from build123d import *

# Parameters (mm, degrees)
SKETCH064_R     = 1.9
POCKET002_DEPTH = 3
SKETCH065_R     = 2
POCKET003_DEPTH = 8


with BuildPart() as part:
    # Sketch063 → Revolution002 (revolve)
    with BuildSketch(Plane.XZ):
        Polygon((5, 13), (5, 0), (16, 0), (16, 3), (8, 3), (8, 13), align=None)
    revolve(axis=Axis((0, 0, 0), (0, 0, 1)))

    # Sketch064 → Pocket002 (cut)
    with BuildSketch(Plane.XY):
        with Locations((-8.485281, 8.485281)):
            Circle(SKETCH064_R)
        with Locations((8.485281, 8.485281)):
            Circle(SKETCH064_R)
        with Locations((8.485281, -8.485281)):
            Circle(SKETCH064_R)
        with Locations((-8.485281, -8.485281)):
            Circle(SKETCH064_R)
    extrude(amount=POCKET002_DEPTH, mode=Mode.SUBTRACT)

    # Sketch065 → Pocket003 (cut, symmetric)
    with BuildSketch(Plane.XZ):
        with Locations((0, 8)):
            Circle(SKETCH065_R)
    extrude(amount=POCKET003_DEPTH, both=True, mode=Mode.SUBTRACT)


with BuildPart() as part_1:
    # Body003 placement: moved
    add(part.part.moved(Location((0, 0, -54.75))))


solid = part_1.part
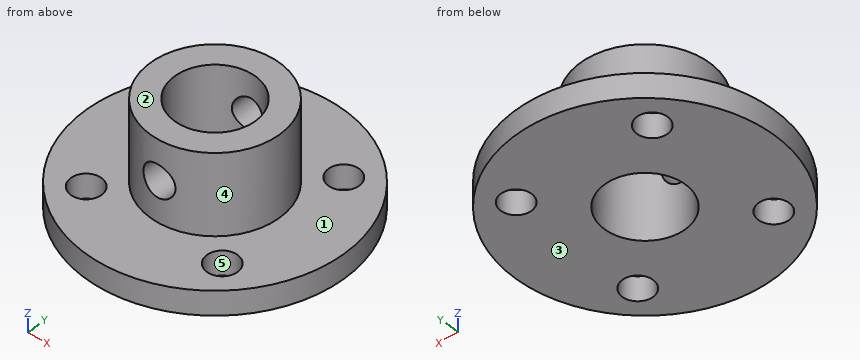
CAD build for the part. Positions are in the model's coordinates, mm. Face numbers are marked on the shaded views. A direction names the side the tool comes from. Round coordinates to 2 decimals unless told otherwise and drop trailing zeros. Write each loop counter-clockwise with the first axis right and the second up, starting at its lowest first coordinate (ties: lowest second). Pieces come first, ordered by that corner, then holes.
(1) Slice it at C-C, the plane z = -47.75. Write the cut outline in (x, y).
(2) Slice it at B-B, the plane y = 1.5. Write the cut outline in (x, z), and give its area (3 significant figures).
(3) 3-axis set-ups, long thin cutter, end or side, ignore diameter. For the marked faces 1 and 2: which of +Z, -Z, +X, -X, +Y, -Y reach the whole face in a straight line?
(4) Slice it at A-A, the plane x = 0. Write the cut outline in (y, z).
(5) Probe line 1 along Z through (x, y) = (0, -7.2); line 2 along X through (y, z) = (-8.5, -52.5); line 3 along Z through (x, y) = (0, 11.5). List the from-to ranges inside material, lowest first.
(6) Slice it at D-D, the plane x = -3.5. Write the cut outline in (y, z), and give its area (3 significant figures).
(7) Drop flat-ended pins along their axis: P1, Ø4, axis at y = -8.5, z = -47, coming from the +X side; P2, Ø4.5, axis at x = 0, z = -46.75, coming from the -Y side; P3, Ø3, axis at x = 8.49, y = 8.49, coming from the +Z side; P4, Ø6, axis at x = 12.5, y = -12, coming from the +Z side. Give the stop position or say it passes through.
(8) Mould opens along X. For the marked faces 3, 4 and 5 say: pulls with the +X half, pulls with the -X half, needs draft (parallel to the pull), parting line crosses it, or undercut.
From the geometry:
1. outline: (-1.73, -7.81) - (-1.73, -4.69) arc R5 cw to (-1.73, 4.69) - (-1.73, 7.81) arc R8 ccw to start; (1.73, -7.81) arc R8 ccw to (1.73, 7.81) - (1.73, 4.69) arc R5 cw to (1.73, -4.69) - close
2. outline: (-15.93, -54.75) - (-4.77, -54.75) - (-4.77, -41.75) - (-7.86, -41.75) - (-7.86, -51.75) - (-15.93, -51.75) - close; (4.77, -54.75) - (15.93, -54.75) - (15.93, -51.75) - (7.86, -51.75) - (7.86, -41.75) - (4.77, -41.75) - close
2. area: 129 mm2
3. face 1: +Z
3. face 2: +Z, +X, -X, +Y, -Y
4. outline: (-16, -54.75) - (-5, -54.75) - (-5, -48.75) - (-8, -48.75) - (-8, -51.75) - (-16, -51.75) - close; (-8, -44.75) - (-5, -44.75) - (-5, -41.75) - (-8, -41.75) - close; (5, -54.75) - (16, -54.75) - (16, -51.75) - (8, -51.75) - (8, -48.75) - (5, -48.75) - close; (5, -44.75) - (8, -44.75) - (8, -41.75) - (5, -41.75) - close
5. line 1: z = -54.75 to -48.75, -44.75 to -41.75
5. line 2: x = -13.56 to -10.39, -6.59 to 6.59, 10.39 to 13.56
5. line 3: z = -54.75 to -51.75
6. outline: (-15.61, -54.75) - (-3.57, -54.75) - (-3.57, -41.75) - (-7.19, -41.75) - (-7.19, -51.75) - (-15.61, -51.75) - close; (3.57, -54.75) - (15.61, -54.75) - (15.61, -51.75) - (7.19, -51.75) - (7.19, -41.75) - (3.57, -41.75) - close
6. area: 145 mm2
7. P1: stops at x = 4.66
7. P2: stops at y = -8
7. P3: passes through
7. P4: stops at z = -51.75
8. face 3: needs draft
8. face 4: parting line crosses it
8. face 5: undercut
